```python
from build123d import *

# Parameters (mm, degrees)
SKETCH2_W           = 1
SKETCH2_H           = 1.0000000000000009
BOSS_EXTRUDE1_DEPTH = 2.5
SNAP_START          = -2.5
SNAP_HOOK2_DEPTH    = 5


# Read off the part's stored shape, not the designer's step: Snap Hook2
with BuildPart() as part:
    # Sketch2 → Boss-Extrude1 (new, symmetric)
    with BuildSketch(Plane.XY):
        with BuildLine():
            Line((-1.319469931058069, 3.8290337033034687), (-3.2925675238278904, 3.8290337033034683))
            ThreePointArc((-3.2925675238278913, 3.829033703303468), (-4.9970052756714, 0.7296836814073608), (-4.25, -2.727636339397171))
            Line((-4.249999999999999, -2.7276363393971716), (-2.9937434759844463, -2.7276363393971716))
            ThreePointArc((-2.9937434759844717, -2.7276363393972467), (-3.9240837129048374, 1.0020314436757887), (-1.319469931058064, 3.829033703303436))
        make_face()
        with BuildLine():
            ThreePointArc((5.05, 0), (4.589660444702355, 2.1065414789019883), (3.29256752382789, 3.8290337033034683))
            Line((3.2925675238278904, 3.829033703303469), (1.3194699310580464, 3.8290337033034687))
            ThreePointArc((1.3194699310580424, 3.8290337033034434), (3.2974500163599956, 2.351451336857189), (4.05, 0))
            ThreePointArc((4.05, -9.9e-16), (3.7767155755853006, -1.4625045166191415), (2.9937434759845, -2.7276363393972156))
            Line((2.993743475984485, -2.7276363393971708), (4.250000000000001, -2.7276363393971708))
            ThreePointArc((4.25, -2.7276363393971708), (4.84587453407535, -1.421267040355192), (5.05, -1.24e-15))
        make_face()
        with BuildLine():
            Line((-2.9937434759844463, -2.7276363393971716), (-4.249999999999999, -2.7276363393971716))
            ThreePointArc((-4.25, -2.727636339397171), (-2.421563181711757, -4.431538305935991), (7.981e-14, -5.05))
            Line((1.49e-15, -5.05), (1.34e-15, -4.05))
            ThreePointArc((-5.11e-14, -4.05), (-1.636394332891877, -3.7046880553265678), (-2.9937434759844717, -2.7276363393972467))
        make_face()
        with BuildLine():
            Line((1.34e-15, -4.05), (1.49e-15, -5.05))
            ThreePointArc((7.981e-14, -5.05), (2.4215631817118264, -4.431538305935953), (4.25, -2.7276363393971708))
            Line((4.250000000000001, -2.7276363393971708), (2.993743475984485, -2.7276363393971708))
            ThreePointArc((2.9937434759845, -2.7276363393972156), (1.6363943328918495, -3.7046880553265797), (-5.11e-14, -4.05))
        make_face()
        with BuildLine():
            ThreePointArc((7.981e-14, -5.05), (-2.421563181711757, -4.431538305935991), (-4.25, -2.727636339397171))
            Line((-4.249999999999999, -2.7276363393971716), (-4.249999999999998, -5.727636339397171))
            Line((-4.249999999999998, -5.727636339397171), (-4.249999999999998, -6.727636339397172))
            Line((-4.249999999999998, -6.727636339397172), (1.78e-15, -6.727636339397172))
            Line((1.73e-15, -6.727636339397171), (1.49e-15, -5.05))
        make_face()
        with Locations((-4.749999999999998, -6.227636339397172)):
            Rectangle(SKETCH2_W, SKETCH2_H)
        with BuildLine():
            ThreePointArc((4.25, -2.7276363393971708), (2.4215631817118264, -4.431538305935953), (7.981e-14, -5.05))
            Line((1.49e-15, -5.05), (1.73e-15, -6.727636339397171))
            Line((1.78e-15, -6.727636339397172), (4.250000000000002, -6.727636339397171))
            Line((4.250000000000002, -6.72763633939717), (4.250000000000002, -5.72763633939717))
            Line((4.250000000000002, -5.72763633939717), (4.250000000000001, -2.7276363393971708))
        make_face()
        Polygon((4.250000000000002, -5.72763633939717), (4.250000000000002, -6.72763633939717), (5.250000000000002, -6.727636339397171), (5.250000000000002, -5.72763633939717), align=None)
    extrude(amount=BOSS_EXTRUDE1_DEPTH, both=True)

    # Snap Hook2 outline → Snap Hook2 (add)
    with BuildSketch(Plane.XY.offset(SNAP_START)):
        Polygon((5.25, -12.027636339), (4.25, -12.027636339), (4.25, -6.727636339), (2.25, -6.727636339), (2.25, -18.027636339), (4.25, -18.027636339), align=None)
    snap_hook2 = extrude(amount=SNAP_HOOK2_DEPTH)

    # Mirror1: Snap Hook2 across plane
    add(snap_hook2.mirror(Plane(origin=(0, 0, 0), x_dir=(0, 0, 1), z_dir=(1, 0, 0))))


solid = part.part
```
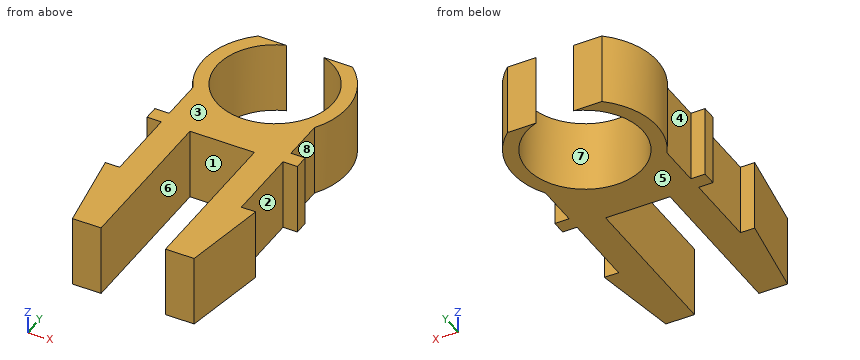
Could you check a few things on this model? Use its own coordinates, in mm. Face numbers are marked on the shaded views. A direction names the side the tool comes from. Coordinates: 2 decimals unless noted, no trailing zeros. Order: outer loops, then holes, each group sorted by start corner. A loop starts at its lowest first (then second) coordinate and runs counter-clockwise, first axis right, second up. Notation, with made-up numbers: M -21.75,78.5 L 29.25,78.5 A33 cw 29.25,111.5 Z; hole C 66.5,63.5 d7. An arc over 180 degrees is marked long. Use a Markdown table: item, result. Add a question column.
Q1. I'm going to push flat-ended pins straight in: pin 1 (2.5 mm diameter, centred on y = -14.5, z = -0.5, fed in from +X); pin 2 (1.5 mm diameter, centred on y = -4.5, z = 0.5, fed in from +X); pin 3 (1.1 mm diameter, centred on x = 4.5, z = -0.5, fed in from +Y). Where does each tip first touch, or does it pass through?
Q2. I want a section at C-C on x = 3.75. List the corners of the cut face in (y, z) for me, then the cut area to 3 significant figures.
Q3. Which directions (+Z, -Z, +X, -X, +Y, -Y) give clear straight access to the entire face, cutting with the end or side of a thin tool? Please do the marked faces 1, 2, 3 and 4.
Q4. I want a section at B-B on z = -0.9. List the corners of the cut face in (x, y) for me.
Q5. I want a section at A-A on y = -9.75. List the corners of the cut face in (x, z) for me, then the cut area to 3 significant figures.
Q6. If I drill on L1, parallel to X at y = 0, z = 1.5; L2, parallel to X at y = -8, z = -0.9; L3, parallel to Y at x = 0, z = -1, over which ranges is the centre line in solid material (lowest first)?
Q7. I want a section at D-D on x = 0. List the corners of the cut face in (y, z) for me.
Q8. We'd pull the mould along X, two halves only. Please class the marked faces 5, 6, 7 and 8: pulls with the +X half, pulls with the -X half, needs draft (parallel to the pull), parting line crosses it, or undercut.
Checked values:
| question | item | result |
|---|---|---|
| 1 | pin 1 | x = 5.05 |
| 1 | pin 2 | x = 4.25 |
| 1 | pin 3 | y = 3.15 |
| 2 | outline | M -18.03,-2.5 L -1.53,-2.5 L -1.53,2.5 L -18.03,2.5 Z; M 1.53,-2.5 L 3.38,-2.5 L 3.38,2.5 L 1.53,2.5 Z |
| 2 | area | 91.8 mm² |
| 3 | face 1 | +Z, -Z, -Y |
| 3 | face 2 | +Z, -Z, +X |
| 3 | face 3 | +Z, +X, -X, +Y, -Y |
| 3 | face 4 | +Z, -Z, -X |
| 4 | outline | M -5.25,-12.03 L -4.25,-18.03 L -2.25,-18.03 L -2.25,-6.73 L 2.25,-6.73 L 2.25,-18.03 L 4.25,-18.03 L 5.25,-12.03 L 4.25,-12.03 L 4.25,-6.73 L 5.25,-6.73 L 5.25,-5.73 L 4.25,-5.73 L 4.25,-2.73 A5.05 ccw 3.29,3.83 L 1.32,3.83 A4.05 cw long -1.32,3.83 L -3.29,3.83 A5.05 ccw -4.25,-2.73 L -4.25,-5.73 L -5.25,-5.73 L -5.25,-6.73 L -4.25,-6.73 L -4.25,-12.03 Z |
| 5 | outline | M -4.25,-2.5 L -2.25,-2.5 L -2.25,2.5 L -4.25,2.5 Z; M 2.25,-2.5 L 4.25,-2.5 L 4.25,2.5 L 2.25,2.5 Z |
| 5 | area | 20.0 mm² |
| 6 | L1 | -5.05 to -4.05, 4.05 to 5.05 |
| 6 | L2 | -4.25 to -2.25, 2.25 to 4.25 |
| 6 | L3 | -6.73 to -4.05 |
| 7 | outline | M -6.73,-2.5 L -4.05,-2.5 L -4.05,2.5 L -6.73,2.5 Z |
| 8 | face 5 | needs draft |
| 8 | face 6 | undercut |
| 8 | face 7 | undercut |
| 8 | face 8 | pulls with the +X half |
